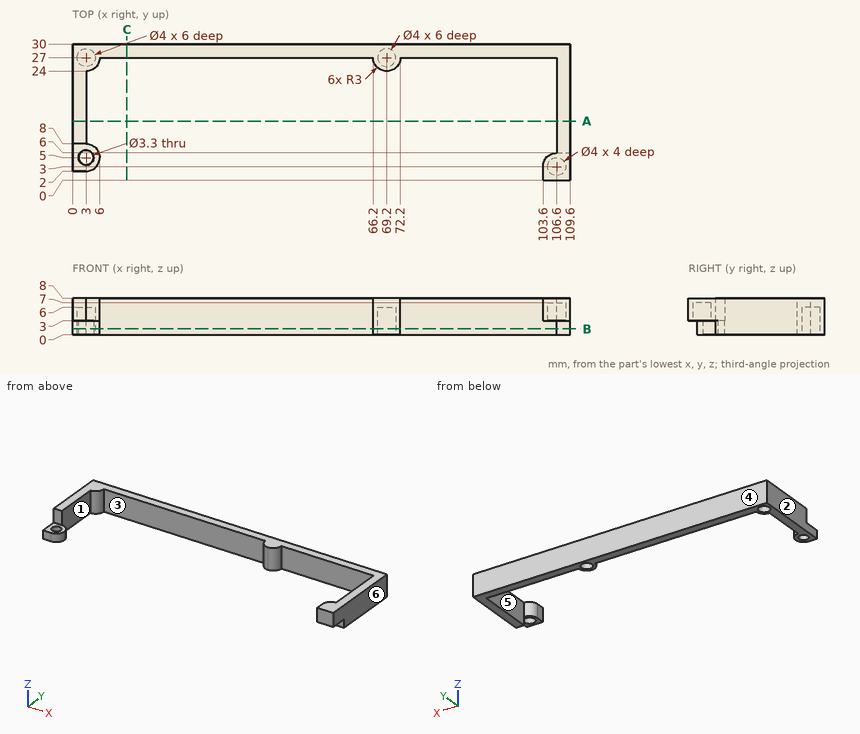
Geometry check sheet. Reference: drawing and pictorial views, mm from the part's lowest x, y, z. A direction names the side the tool comes from. Give positions to 0.01 mm unless a question says otherwise; leave off trailing zeros. Loops run counter-clockwise (first coordinate to the right, second up) from the corner with the lowest first, then second, coordinate; pieces in that order, holes last. Notation, with made-up numbers: (-12, -9.5) - (-5, -9.5) arc R22 ccw to (-5, 25.5) - close; hole circle Ø2 at (8.5, -5.5). An arc over 180 degrees is marked (long way). Use CSV: the item, a comma, the result in double quotes. Start each with the question number.
Q1. Access from +Z, -Z, +X, -X, +Y, -Y to the whole of each face (thin tool, end or side, straight path). Record for the marked faces 1, 2 and 3.
Q2. Go/stop test with flat-tipped pins: pin 1 Ø0.9 at (x, z) = (108.5, 1.5) entering from -Y; pin 2 Ø3.5 at (x, z) = (2, 2) entering from -Y; pin 3 Ø0.9 at (y, z) = (2, 6) entering from -X; pin 4 Ø3 at (x, y) = (3, 5) entering from +Z. Record where each tip stops, or that it passes through.
Q3. Release check for a two-part mould opening along X. For the marked faces 4, 5 and 6 record: +X half, -X half, draft (parallel to the pull), parting line (faces both ways), or undercut.
Q4. Scan lines: probe 1 along X at (y, z) = (21.75, 7.5); probe 2 along X at (y, z) = (5, 1.25); probe 3 along X at (y, z) = (26.5, 6.25). Record each from-to range of solid material in increasing order. Write a range as from..to.
Q5. Section check B-B, the plane z = 1.25. Count the separate pieces of the cut face and the enclosed holes in it.
Q6. Section check A-A, the plane y = 13. Record the cut outline in (x, z).
Q7. Section check C-C, the plane x = 12. Record the cut outline in (y, z).
Findings below:
1,face 1,"+Z, -Z"
1,face 2,"+Z, -Z, -X, +Y, -Y"
1,face 3,"+Z, -Z, -Y"
2,pin 1,"stops at y = 6"
2,pin 2,"stops at y = 2"
2,pin 3,"stops at x = 103.6"
2,pin 4,"passes through"
3,face 4,"draft"
3,face 5,"undercut"
3,face 6,"+X half"
4,probe 1,"x = 0..3, 106.6..109.6"
4,probe 2,"x = 0..1.35, 4.65..6"
4,probe 3,"x = 0..5.96, 66.24..72.16, 106.6..109.6"
5,separate pieces,"1"
5,enclosed holes,"3"
6,outline,"(0, 0) - (3, 0) - (3, 8) - (0, 8) - close; (106.6, 0) - (109.6, 0) - (109.6, 8) - (106.6, 8) - close"
7,outline,"(27, 0) - (30, 0) - (30, 8) - (27, 8) - close"
